Work out the finished part from the listing and answer in its coordinate system (mm). Face numbers are marked on the shaded views. A direction names the side the tool comes from. Give positions to 0.01 mm unless a question says otherwise; leave off trailing zeros. Loops run counter-clockwise (first coordinate to the right, second up) from the corner with the lowest first, then second, coordinate; pieces in that order, holes last. Notation, with made-up numbers: M -14,-24.75 L 40,-24.75 A13 cw 40,-2.75 Z; hole C -4.5,-26 d8. An arc over 180 degrees is marked long. Write item = value, one per line. Start each with the question number.
1. Consider L1, parallel to X at y = 54, z = 3.25; L2, parallel to X at y = 35.5, z = 6.5; L3, parallel to X at y = 56.5, z = 1.5. Determine where each line is inside the solid, lowest interval first. Write a range as [from, to].
2. Section A-A on y = 25 is taken. Determine the outline of the cut face in (x, z).
3. Section B-B on x = 121.5 is taken. Determine the outline of the cut face in (y, z).
4. For the marked faces 1, 2 and 3, determine the directions among +Z, -Z, +X, -X, +Y, -Y from which every point of the face is accessible in a straight line to the end or side of a thin tool.
5. Flat-ended cylindrical pins translate along their axes: pin 1 Ø10 at (y, z) = (13.5, 11.5) entering from -X; pin 2 Ø3.5 at (x, z) = (96, 2) entering from -Y; pin 3 Ø6 at (x, y) = (81, 49.5) entering from +Z. Find the tip coordinate at first contact, or state that the pin passes through.
6. Section C-C on z = 3 is taken. Determine the outline of the cut face in (x, y).
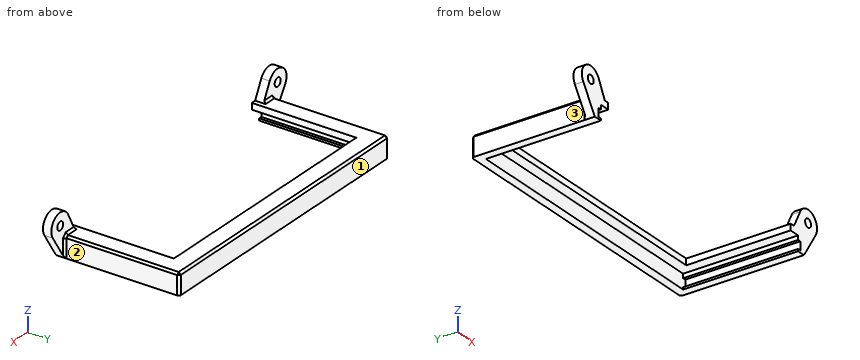
```python
from build123d import *

# Parameters (mm, degrees)
SKETCH1_W           = 141
SKETCH1_H           = 59
BOSS_EXTRUDE1_DEPTH = 10
SKETCH2_W           = 133
SKETCH2_H           = 55
CUT_EXTRUDE1_DEPTH  = 7
SKETCH3_W           = 123
SKETCH3_H           = 50
CUT_EXTRUDE2_DEPTH  = 7
SKETCH4_W           = 1.5
SKETCH4_H           = 4
CUT_EXTRUDE3_DEPTH  = 55
SKETCH5_R           = 2
BOSS_EXTRUDE2_DEPTH = 4
CHAMFER1_SIZE       = 1


with BuildPart() as part:
    # Sketch1 → Boss-Extrude1 (new body)
    with BuildSketch(Plane.XY):
        with Locations((70.5, 29.5)):
            Rectangle(SKETCH1_W, SKETCH1_H)
    extrude(amount=BOSS_EXTRUDE1_DEPTH)

    # Sketch2 → Cut-Extrude1 (cut)
    with BuildSketch(Plane(origin=(0, 0, 0), x_dir=(-1, 0, 0), z_dir=(0, 0, -1))):
        with Locations((-70.5, 27.5)):
            Rectangle(SKETCH2_W, SKETCH2_H)
    extrude(amount=-CUT_EXTRUDE1_DEPTH, mode=Mode.SUBTRACT)

    # Sketch3 → Cut-Extrude2 (cut)
    with BuildSketch(Plane(origin=(0, 0, 7), x_dir=(-1, 0, 0), z_dir=(0, 0, -1))):
        with Locations((-70.5, 25)):
            Rectangle(SKETCH3_W, SKETCH3_H)
    extrude(amount=-CUT_EXTRUDE2_DEPTH, mode=Mode.SUBTRACT)

    # Sketch4 → Cut-Extrude3 (cut)
    with BuildSketch(Plane(origin=(0, 0, 0), x_dir=(-1, 0, 0), z_dir=(0, -1, 0))):
        with Locations((-3.25, -3)):
            Rectangle(SKETCH4_W, SKETCH4_H)
        with Locations((-137.75, -3)):
            Rectangle(SKETCH4_W, SKETCH4_H)
    extrude(amount=-CUT_EXTRUDE3_DEPTH, mode=Mode.SUBTRACT)

    # Sketch5 → Boss-Extrude2 (add)
    with BuildSketch(Plane(origin=(0, 0, 0), x_dir=(-1, 0, 0), z_dir=(0, -1, 0))):
        with BuildLine():
            Line((-2.565492231, -18.088154896), (-6.758248996, -10))
            Line((-6.758248996, -10), (0, -10))
            Line((0, -10), (0, 0))
            Line((0, 0), (7.800562775, -12.070115644))
            ThreePointArc((7.800562775, -12.070115644), (5.773784886, -20.515765997), (-2.565492231, -18.088154896))
        make_face()
        with Locations((2.761331332, -15.326823563)):
            Circle(SKETCH5_R, mode=Mode.SUBTRACT)
        with BuildLine():
            Line((-141, -10), (-134.241751004, -10))
            Line((-134.241751004, -10), (-138.434507769, -18.088154896))
            ThreePointArc((-138.434507769, -18.088154896), (-146.773784886, -20.515765997), (-148.800562775, -12.070115644))
            Line((-148.800562775, -12.070115644), (-141, 0))
            Line((-141, 0), (-141, -10))
        make_face()
        with Locations((-143.761331332, -15.326823563)):
            Circle(SKETCH5_R, mode=Mode.SUBTRACT)
    extrude(amount=-BOSS_EXTRUDE2_DEPTH)

    # Chamfer1
    chamfer1_edges = [part.edges().sort_by_distance(p)[0] for p in [
        (70.5, 59, 10),
        (0, 31.5, 10),
        (0, 59, 5),
        (141, 59, 5),
        (3.379124498, 4, 10),
        (0, 4, 5),
        (141, 31.5, 10),
        (141, 4, 5),
        (137.620875502, 4, 10),
    ]]
    chamfer(chamfer1_edges, length=CHAMFER1_SIZE)


solid = part.part
```
Verdict:
q1.L1 = [0, 2.5], [138.5, 141]
q1.L2 = [0, 4], [137, 141]
q1.L3 = [0, 141]
q2.outline = M 0,0 L 4,0 L 4,1 L 2.5,1 L 2.5,5 L 4,5 L 4,7 L 9,7 L 9,10 L 1,10 L 0,9 Z; M 132,7 L 137,7 L 137,5 L 138.5,5 L 138.5,1 L 137,1 L 137,0 L 141,0 L 141,9 L 140,10 L 132,10 Z
q3.outline = M 50,7 L 55,7 L 55,0 L 59,0 L 59,9 L 58,10 L 50,10 Z
q4.face_1 = +Z, -Z, +X, -X, +Y
q4.face_2 = +Z, -Z, +X, +Y
q4.face_3 = +Z, -Z, -X, +Y
q5.pin_1 = 0
q5.pin_2 = 55
q5.pin_3 = 10
q6.outline = M -1.94,0 L 2.5,0 L 2.5,55 L 138.5,55 L 138.5,0 L 142.94,0 L 142.94,4 L 142,4 L 141,5 L 141,58 L 140,59 L 1,59 L 0,58 L 0,5 L -1,4 L -1.94,4 Z
